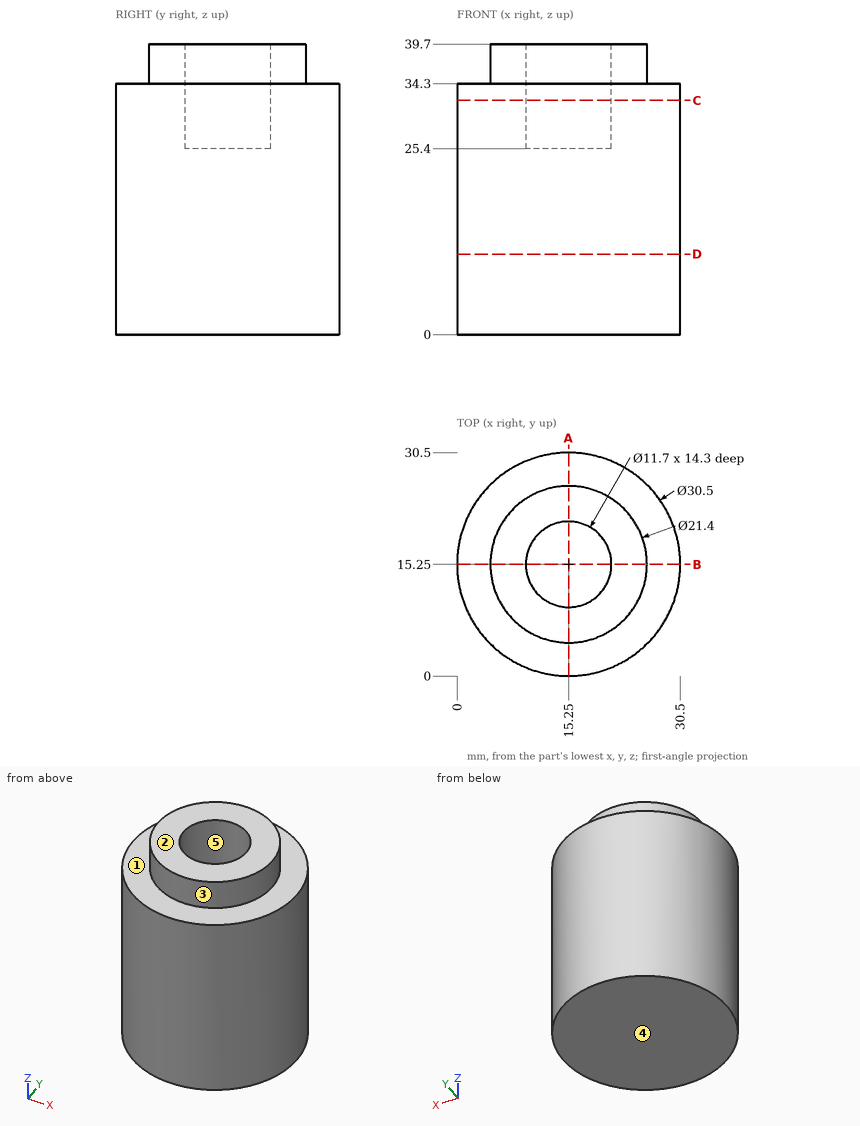
Geometry: see drawing. Coordinates: mm, zero at the bounding-box minimum. A direction names the side the tool comes from. Round coordinates to 2 decimals unless told otherwise and drop trailing zeros. Loops run counter-clockwise (first coordinate to the right, second up) from the corner with the lowest first, then second, coordinate; pieces in that order, holes last. Notation, with made-up numbers: M 36,77.25 L 57,77.25 A22 cw 57,97.25 Z; hole C -20,24.25 d8. An arc over 180 degrees is marked long. Use a Markdown table: item, result. Add a question column.
1. Set-up query: the marked faces 1 and 2. Return all of +Z, -Z, +X, -X, +Y, -Y with unobstructed straight access to the full face (end or side cutting, diameter ignored); none if empty.
2. Cut plane C-C, the plane z = 32. Output: boundary loops of the cut face in (x, y).
3. Cut plane A-A, the plane x = 15.25. Output: boundary loops of the cut face in (y, z).
4. Ray query, line 1 along Y through (x, z) = (15, 32); line 2 along Z through (x, y) = (24, 4); line 3 along X through (y, z) = (20.5, 27.5). Return the intervals inside material, ascending. Write a range as [from, to].
5. Cut plane D-D, the plane z = 11. Output: boundary loops of the cut face in (x, y).
6. Contact query for flat-ended pins moving along their axis: pin 1 (1 mm diameter, centred on x = 8.5, z = 5, fed in from -Y); pin 2 (1.5 mm diameter, centred on y = 21.5, z = 28.5, fed in from +X); pin 3 (4 mm diameter, centred on x = 19, z = 33, fed in from +Y); pin 4 (8 mm diameter, centred on x = 4.5, y = 25, fed in from -Z). Output: stop coordinate, or through.
7. Pull-direction query (Y, two-part tool) for the marked faces 3, 4 and 5; classes: +Y half, -Y half, draft (parallel to the pull), parting line (faces both ways), or undercut.
Solution:
| question | item | result |
|---|---|---|
| 1 | face 1 | +Z |
| 1 | face 2 | +Z, +X, -X, +Y, -Y |
| 2 | outline | C 15.25,15.25 d30.5; hole C 15.25,15.25 d11.7 |
| 3 | outline | M 0,0 L 30.5,0 L 30.5,34.3 L 25.95,34.3 L 25.95,39.7 L 21.1,39.7 L 21.1,25.4 L 9.4,25.4 L 9.4,39.7 L 4.55,39.7 L 4.55,34.3 L 0,34.3 Z |
| 4 | line 1 | y = [0, 9.41], [21.09, 30.5] |
| 4 | line 2 | z = [0, 34.3] |
| 4 | line 3 | x = [0.93, 12.67], [17.83, 29.57] |
| 5 | outline | C 15.25,15.25 d30.5 |
| 6 | pin 1 | stops at y = 1.34 |
| 6 | pin 2 | stops at x = 29.47 |
| 6 | pin 3 | stops at y = 30.4 |
| 6 | pin 4 | stops at z = 0 |
| 7 | face 3 | parting line |
| 7 | face 4 | draft |
| 7 | face 5 | undercut |
